```python
from build123d import *

# Parameters (mm, degrees)
SKETCH_1_R          = 7.55
EXTRUDE_1_DEPTH     = 3.5
CUT_EXTRUDE_1_DEPTH = 27.5


with BuildPart() as part:
    # Эскиз1 → Бобышка-Вытянуть1 (new body)
    with BuildSketch(Plane.XY):
        Polygon((0, 11.75), (-10.175798494, 5.875), (-10.175798494, -5.875), (0, -11.75), (10.175798494, -5.875), (10.175798494, 5.875), align=None)
        Circle(SKETCH_1_R, mode=Mode.SUBTRACT)
    extrude(amount=EXTRUDE_1_DEPTH)

    # Эскиз3 → Вырез-Повернуть2 (revolve, cut)
    with BuildSketch(Plane(origin=(0, 0, 0), x_dir=(0, 0, -1), z_dir=(1, 0, 0))):
        with BuildLine():
            Line((-2.149262527, 11.75), (-3.5, 11.75))
            Line((-3.5, 11.75), (-3.5, 10.15))
            ThreePointArc((-3.5, 10.15), (-3.06988498, 11.157045866), (-2.149262527, 11.75))
        make_face()
    revolve(axis=Axis((0, 0, 10.349500572), (0, 0, -1)), mode=Mode.SUBTRACT)

    # Эскиз4 → Вырез-Вытянуть1 (cut)
    with BuildSketch(Plane.XY.offset(20)):
        Polygon((-4.438380194, 9.1875), (-5.7374183, 8.4375), (-5.4374183, 7.917884758), (-4.138380194, 8.667884758), align=None)
    extrude(amount=-CUT_EXTRUDE_1_DEPTH, mode=Mode.SUBTRACT)


solid = part.part
```
Geometry check sheet. Reference: the model listing, model coordinates, mm. Round coordinates to 2 decimals unless told otherwise and drop trailing zeros. Return JSON: item names as keys, results as strings. Group by question number.
(1) Mould release check, pull along Y, two halves, no side actions. Record for faces 1 (the face through (-4.797, 8.288, 1.774)), 2 (the face through (5.02, -8.85, 1.72)), 3 (the face through (-10.176, 0, 2)): pulls with the +Y half, pulls with the -Y half, needs draft (parallel to the pull), parting line crosses it, or undercut.
(2) Scan lines: line 1 along X through (y, z) = (-7, 0.5); line 2 along X through (y, z) = (5.5, 3); line 3 along Y through (x, z) = (-1.75, 1.45). Record each from-to range of solid material in increasing order. Write a range as [from, to].
(3) Go/stop test with flat-tipped pins: pin 1 (8 mm diameter, centred on x = 4, y = 6, fed in from +Z); pin 2 (1.5 mm diameter, centred on x = 1.5, z = 0.5, fed in from -Y). Record where each tip stops, or that it passes through.
Data:
{
 "1": {"face 1": "undercut", "face 2": "pulls with the -Y half", "face 3": "needs draft"},
 "2": {"line 1": "[-8.23, -2.83], [2.83, 8.23]", "line 2": "[-9.8, -5.17], [5.17, 9.8]", "line 3": "[-10.74, -7.34], [7.34, 10.74]"},
 "3": {"pin 1": "z = 3.5", "pin 2": "y = -11.32"}
}
